from build123d import *

# Parameters (mm, degrees)
SKETCH1_W                   = 160
SKETCH1_H                   = 140
LID_EXTRUDE_DEPTH           = 20
SKETCH3_W                   = 5
SKETCH3_H                   = 95
LOCATION_BAR_EXTRUDE_DEPTH  = 10
M6_TAPPED_HOLE1_D           = 5
M6_TAPPED_HOLE1_CSINK_D     = 6.05
M6_TAPPED_HOLE1_CSINK_ANGLE = 90
SKETCH6_R                   = 16
MOTOR_HOLE_CUT_DEPTH        = 3.15
FILLET2_R                   = 1
SKETCH7_R                   = 7.5
CUT_EXTRUDE1_DEPTH          = 111.453610172
CUT_EXTRUDE3_START          = -10
SKETCH9_R                   = 7.5
CUT_EXTRUDE3_DEPTH          = 10


with BuildPart() as part:
    # Sketch1 → LID_EXTRUDE (new body)
    with BuildSketch(Plane(origin=(0, 0, 0), x_dir=(1, 0, 0), z_dir=(0, 1, 0))):
        Rectangle(SKETCH1_W, SKETCH1_H)
    extrude(amount=LID_EXTRUDE_DEPTH)

    # Sketch3 → LOCATION_BAR_EXTRUDE (add)
    with BuildSketch(Plane(origin=(0, 20, 0), x_dir=(1, 0, 0), z_dir=(0, 1, 0))):
        with Locations((-57.5, 0)):
            Rectangle(SKETCH3_W, SKETCH3_H)
        with Locations((57.5, 0)):
            Rectangle(SKETCH3_W, SKETCH3_H)
    extrude(amount=LOCATION_BAR_EXTRUDE_DEPTH)

    # M6 Tapped Hole1 (through all)
    with Locations(Plane(origin=(0, 0, 55), x_dir=(0, 0, -1), z_dir=(0, -1, 0))):
        with Locations((0, 0), (55, -65)):
            m6_tapped_hole1 = CounterSinkHole(M6_TAPPED_HOLE1_D / 2, M6_TAPPED_HOLE1_CSINK_D / 2, counter_sink_angle=M6_TAPPED_HOLE1_CSINK_ANGLE)

    # Mirror1: M6 Tapped Hole1 across plane
    add(m6_tapped_hole1.mirror(Plane(origin=(0, 0, 0), x_dir=(0, 0, 1), z_dir=(1, 0, 0))), mode=Mode.SUBTRACT)

    # Mirror1 at the second plane: M6 Tapped Hole1 across plane
    add(m6_tapped_hole1.mirror(Plane.XY), mode=Mode.SUBTRACT)

    # Sketch6 → MOTOR_HOLE_CUT (cut)
    with BuildSketch(Plane.XZ):
        with Locations(Location((15, 0, 0), (0, 0, 270))):
            Circle(SKETCH6_R)
    extrude(amount=-MOTOR_HOLE_CUT_DEPTH, mode=Mode.SUBTRACT)

    # Fillet2
    fillet2_edges = [part.edges().sort_by_distance(p)[0] for p in [
        (80, 20, 0),
        (0, 20, -70),
        (-80, 20, 0),
        (0, 0, -70),
        (80, 0, 0),
        (0, 0, 70),
        (-80, 0, 0),
        (0, 20, 70),
    ]]
    fillet(fillet2_edges, radius=FILLET2_R)

    # Sketch7 → Cut-Extrude1 (cut, through all)
    with BuildSketch(Plane.XZ):
        with Locations(Location((15, 0, 0), (0, 0, 270))):
            Circle(SKETCH7_R)
    extrude(amount=-CUT_EXTRUDE1_DEPTH, mode=Mode.SUBTRACT)

    # Sketch9 → Cut-Extrude3 (cut)
    with BuildSketch(Plane.XZ.offset(CUT_EXTRUDE3_START)):
        with Locations(Location((-15, 0, 0), (0, 0, 90))):
            Circle(SKETCH9_R)
    extrude(amount=-CUT_EXTRUDE3_DEPTH, mode=Mode.SUBTRACT)


solid = part.part
Geometry check sheet. Reference: the model listing, model coordinates, mm. A direction names the side the tool comes from. Round coordinates to 2 decimals unless told otherwise and drop trailing zeros. Write each loop counter-clockwise with the first axis right and the second up, starting at its lowest first coordinate (ties: lowest second). Pieces come first, ordered by that corner, then holes. Notation, with made-up numbers: (67.5, 7.5) -> (86.5, 7.5) arc R20 cw to (86.5, 36.5) -> close; hole circle Ø10 at (-26.75, -11). An arc over 180 degrees is marked (long way). One line per item, written item: value. Start each with the question number.
(1) Cross-section at A-A, the plane x = -65. Record the cut outline in (y, z) (3 decimals).
(2) Go/stop test with flat-tipped pins: pin 1 Ø12 at (x, z) = (-18, 0.5) entering from +Y; pin 2 Ø2 at (y, z) = (27, 23.5) entering from -X; pin 3 Ø5.5 at (x, y) = (58.5, 23.5) entering from +Z. Record where each tip stops, or that it passes through.
(3) Cross-section at B-B, the plane z = 55. Record the cut outline in (x, y) (3 decimals), and give its area (3 significant figures).
(4) Cross-section at D-D, the plane y = 24. Record the cut outline in (x, z).
(5) Access from +Z, -Z, +X, -X, +Y, -Y to the whole of each face (thin tool, end or side, straight path). Record for faces 1 (the flat face through (-58, 25, 47.5)), 2 (the cylindrical face through (-21.324, 14.93, 4.032)), 3 (the cylindrical face through (-0.62, 1.55, 3.47)), 4 (the flat face through (-58, 25, -47.5)), 5 (the flat face through (55, 25, 1)).
(6) Scan lines: line 1 (X direction, y = 16.25, z = 0); line 2 (X direction, y = 7.75, z = 0); line 3 (Z direction, x = 0, y = 13). Record each from-to range of solid material in increasing order. Write a range as [from, to].
(7) Cross-section at C-C, the plane y = 14.5. Record the cut outline in (x, z), and give its area (3 significant figures).
(8) Draft check along X on faces 6 (the flat face through (60, 25, 1)), 7 (the flat face through (-55, 25, 1)), 8 (the cylindrical face through (-0.96, 10.4, 57.31)), 9 (the flat face through (-1, 10, -70)). Enter one of: +X half, -X half, draft (parallel to the pull), parting line (faces both ways), or undercut.
Answer:
1. outline: (0, -69) arc R1 ccw to (1, -70) -> (19, -70) arc R1 ccw to (20, -69) -> (20, -2.5) -> (0.525, -2.5) -> (0, -3.025) -> close; (0, 3.025) -> (0.525, 2.5) -> (20, 2.5) -> (20, 69) arc R1 ccw to (19, 70) -> (1, 70) arc R1 ccw to (0, 69) -> close
2. pin 1: y = 20
2. pin 2: x = -60
2. pin 3: z = 47.5
3. outline: (-80, 1) arc R1 ccw to (-79, 0) -> (-3.025, 0) -> (-2.5, 0.525) -> (-2.5, 20) -> (-79, 20) arc R1 ccw to (-80, 19) -> close; (2.5, 0.525) -> (3.025, 0) -> (79, 0) arc R1 ccw to (80, 1) -> (80, 19) arc R1 ccw to (79, 20) -> (2.5, 20) -> close
3. area: 3,100 mm²
4. outline: (-60, -47.5) -> (-55, -47.5) -> (-55, 47.5) -> (-60, 47.5) -> close; (55, -47.5) -> (60, -47.5) -> (60, 47.5) -> (55, 47.5) -> close
5. face 1: +Z, +X, -X, +Y
5. face 2: +Y
5. face 3: -Y
5. face 4: -Z, +X, -X, +Y
5. face 5: +Z, -Z, +Y
6. line 1: [-80, -67.5], [-62.5, -22.5], [-7.5, 7.5], [22.5, 62.5], [67.5, 80]
6. line 2: [-80, -67.5], [-62.5, 7.5], [22.5, 62.5], [67.5, 80]
6. line 3: [-70, -57.5], [-52.5, 52.5], [57.5, 70]
7. outline: (-80, -70) -> (80, -70) -> (80, 70) -> (-80, 70) -> close; hole circle Ø5 at (-65, 0); hole circle Ø15 at (-15, 0); hole circle Ø5 at (0, -55); hole circle Ø5 at (0, 55); hole circle Ø15 at (15, 0); hole circle Ø5 at (65, 0)
7. area: 22,000 mm²
8. face 6: +X half
8. face 7: undercut
8. face 8: undercut
8. face 9: draft
